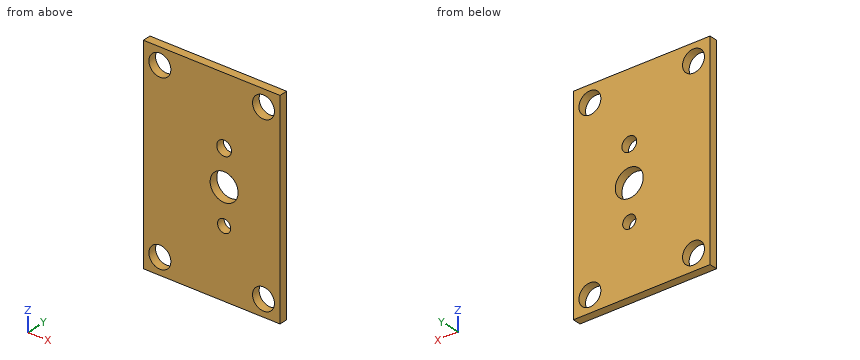
```python
from build123d import *

# Parameters (mm, degrees)
SKETCH1_W           = 25
SKETCH1_H           = 50
SKETCH1_R           = 3.375
BOSS_EXTRUDE1_DEPTH = 2
SKETCH2_W           = 50
SKETCH2_H           = 2
BOSS_EXTRUDE2_DEPTH = 8
SKETCH3_W           = 8
SKETCH3_H           = 50
BOSS_EXTRUDE3_DEPTH = 42
SKETCH4_R           = 2.65
CUT_EXTRUDE1_DEPTH  = 3.3
SKETCH5_R           = 5.802370205
CUT_EXTRUDE2_DEPTH  = 9
FILLET2_R           = 1
SKETCH6_R           = 12.7
BOSS_EXTRUDE4_DEPTH = 2
FILLET4_R           = 1
SKETCH8_R           = 1.589780168
SKETCH8_R_2         = 1.777428262
CUT_EXTRUDE3_DEPTH  = 10
SKETCH9_W           = 8
SKETCH9_H           = 42
CUT_EXTRUDE4_DEPTH  = 68.79439129
SKETCH10_W          = 33.517939775
SKETCH10_H          = 7.212330843
CUT_EXTRUDE5_DEPTH  = 55


with BuildPart() as part:
    # Sketch1 → Boss-Extrude1 (new body)
    with BuildSketch(Plane(origin=(0, 0, 0), x_dir=(1, 0, 0), z_dir=(0, 1, 0))):
        with Locations((2.276951673, 11.384758364)):
            Rectangle(SKETCH1_W, SKETCH1_H)
        with Locations(Location((1.276951673, 11.384758364, 0), (0, 0, 270))):
            Circle(SKETCH1_R, mode=Mode.SUBTRACT)
    extrude(amount=BOSS_EXTRUDE1_DEPTH)

    # Sketch2 → Boss-Extrude2 (add)
    with BuildSketch(Plane.ZY.offset(10.223048327)):
        with Locations((-11.384758364, 1)):
            Rectangle(SKETCH2_W, SKETCH2_H)
    extrude(amount=BOSS_EXTRUDE2_DEPTH)

    # Sketch3 → Boss-Extrude3 (add)
    with BuildSketch(Plane.XZ):
        with Locations((-14.223048327, -11.384758364)):
            Rectangle(SKETCH3_W, SKETCH3_H)
    extrude(amount=BOSS_EXTRUDE3_DEPTH)

    # Sketch4 → Cut-Extrude1 (cut)
    with BuildSketch(Plane(origin=(0, 2, 0), x_dir=(1, 0, 0), z_dir=(0, 1, 0))):
        with Locations(Location((-14.223048327, 32.384758364, 0), (0, 0, 270))):
            Circle(SKETCH4_R)
        with Locations(Location((-14.223048327, -9.615241636, 0), (0, 0, 270))):
            Circle(SKETCH4_R)
    cut_extrude1 = extrude(amount=-CUT_EXTRUDE1_DEPTH, mode=Mode.SUBTRACT)

    # Mirror1: Cut-Extrude1 across plane
    add(cut_extrude1.mirror(Plane.ZX.offset(-20)), mode=Mode.SUBTRACT)

    # Sketch5 → Cut-Extrude2 (cut)
    with BuildSketch(Plane.ZY.offset(18.223048327)):
        with Locations((-11.836279124, -21)):
            Circle(SKETCH5_R)
    extrude(amount=-CUT_EXTRUDE2_DEPTH, mode=Mode.SUBTRACT)

    # Fillet2
    fillet2_edges = [part.edges().sort_by_distance(p)[0] for p in [
        (-10.223048327, -21, -17.638649329),
    ]]
    fillet(fillet2_edges, radius=FILLET2_R)

    # Mirror2: Cut-Extrude1 across plane
    add(cut_extrude1.mirror(Plane.ZY.offset(1.723048327)), mode=Mode.SUBTRACT)

    # Sketch6 → Boss-Extrude4 (add)
    with BuildSketch(Plane(origin=(0, 2, 0), x_dir=(1, 0, 0), z_dir=(0, 1, 0))):
        with BuildLine():
            Line((14.776951673, 5.567542535), (14.776951673, 17.201974193))
            ThreePointArc((14.776951673, 17.201974193), (-13.423048327, 11.384758364), (14.776951673, 5.567542535))
        make_face()
        with Locations(Location((1.276951673, 11.384758364, 0), (0, 0, 270))):
            Circle(SKETCH6_R, mode=Mode.SUBTRACT)
    extrude(amount=BOSS_EXTRUDE4_DEPTH)

    # Fillet4
    # the kernel refuses this fillet: 1 mm, written as the material it takes off along each edge
    with BuildSketch(Plane(origin=(14.776951673, 4, -3.067542535), x_dir=(0, -1, 0), z_dir=(0, 0, -1))) as fillet4_piece_1:
        with BuildLine():
            CenterArc((FILLET4_R, FILLET4_R), FILLET4_R, 180, 90)
            Line((0, FILLET4_R), (0, 0))
            Line((0, 0), (FILLET4_R, 0))
        make_face()
    extrude(amount=16.634431658, mode=Mode.SUBTRACT)

    # Sketch8 → Cut-Extrude3 (cut)
    with BuildSketch(Plane(origin=(0, 2, 0), x_dir=(1, 0, 0), z_dir=(0, 1, 0))):
        with Locations(Location((1.276951673, 19.884758364, 0), (0, 0, 270))):
            Circle(SKETCH8_R)
        with Locations(Location((1.276951673, 2.884758364, 0), (0, 0, 270))):
            Circle(SKETCH8_R_2)
    extrude(amount=-CUT_EXTRUDE3_DEPTH, mode=Mode.SUBTRACT)

    # Sketch9 → Cut-Extrude4 (cut, through all)
    with BuildSketch(Plane.XY.offset(13.615241636)):
        with Locations((-14.223048327, -21)):
            Rectangle(SKETCH9_W, SKETCH9_H)
    extrude(amount=-CUT_EXTRUDE4_DEPTH, mode=Mode.SUBTRACT)

    # Sketch10 → Cut-Extrude5 (cut)
    with BuildSketch(Plane.XY.offset(13.615241636)):
        with Locations((-1.464078439, 5.606165422)):
            Rectangle(SKETCH10_W, SKETCH10_H)
    extrude(amount=-CUT_EXTRUDE5_DEPTH, mode=Mode.SUBTRACT)


solid = part.part
```
Here's how the part is built. I have some questions about the finished solid (model axes, mm). Give positions to 0.01 mm unless a question says otherwise; leave off trailing zeros. Write each loop counter-clockwise with the first axis right and the second up, starting at its lowest first coordinate (ties: lowest second). Pieces come first, ordered by that corner, then holes. Notation, with made-up numbers: (-6, -20.5) -> (13, -20.5) arc R21 ccw to (13, 13.5) -> close; hole circle Ø6 at (59, 44). An arc over 180 degrees is marked (long way). Use one line per item in the form item = value.
1) Suppose I cut it at B-B (z = -9.5). Please give me the cut outline in (x, y).
Verdict:
outline = (-18.22, 0) -> (-1.52, 0) -> (-1.52, 2) -> (-18.22, 2) -> close; (4.08, 0) -> (14.78, 0) -> (14.78, 2) -> (4.08, 2) -> close
2) Suppose I cut it at C-C (z = -2). Please give me the cut outline in (x, y).
Verdict:
outline = (-18.22, 0) -> (-0.26, 0) -> (-0.26, 2) -> (-18.22, 2) -> close; (2.82, 0) -> (14.78, 0) -> (14.78, 2) -> (2.82, 2) -> close
3) If I drill on L1, parallel to Z at x = 11, y = 1.25; L2, parallel to Z at x = -15, y = 0.75; L3, parallel to X at y = 0.4, z = 9, over which ranges is the centre line in solid material (lowest first)? Write a range as [from, to].
Verdict:
L1 = [-36.38, -35.03], [-29.74, 6.97], [12.26, 13.62]
L2 = [-36.38, -34.92], [-29.85, 7.08], [12.15, 13.62]
L3 = [-18.22, -16.8], [-11.65, 8.2], [13.35, 14.78]
4) Suppose I cut it at A-A (y = 0.5). Please give me the cut outline in (x, z) (3 decimals).
Verdict:
outline = (-18.223, -36.385) -> (14.777, -36.385) -> (14.777, 13.615) -> (-18.223, 13.615) -> close; hole circle Ø5.3 at (-14.223, -32.385); hole circle Ø5.3 at (-14.223, 9.615); hole circle Ø6.75 at (1.277, -11.385); hole circle Ø3.555 at (1.277, -2.885); hole circle Ø3.18 at (1.277, -19.885); hole circle Ø5.3 at (10.777, -32.385); hole circle Ø5.3 at (10.777, 9.615)
5) I'm going to push flat-ended pins straight in: pin 1 (4 mm diameter, centred on x = 10.78, z = -32.38, fed in from +Y); pin 2 (8.5 mm diameter, centred on x = -14.22, z = 9.62, fed in from -Y). Where does each tip first touch, or does it pass through?
Verdict:
pin_1 = through
pin_2 = 0
